from build123d import *

# Parameters (mm, degrees)
BOSS_EXTRUDE1_DEPTH     = 8.255
SKETCH2_R               = 9.525
BOSS_EXTRUDE2_DEPTH     = 0.635
CUT_EXTRUDE1_DEPTH      = 17.139496584
CUT_EXTRUDE1_DEPTH_BACK = 17.139496584
SKETCH3_R               = 2.159
FILLET1_R               = 2.54


with BuildPart() as part:
    # Sketch1 → Boss-Extrude1 (new body)
    with BuildSketch(Plane(origin=(0, 0, 0), x_dir=(1, 0, 0), z_dir=(0, 1, 0))):
        Polygon((7.18570145, 0), (3.592850725, 6.223), (-3.592850725, 6.223), (-7.18570145, 0), (-3.592850725, -6.223), (3.592850725, -6.223), align=None)
    extrude(amount=BOSS_EXTRUDE1_DEPTH)

    # Sketch2 → Boss-Extrude2 (add)
    with BuildSketch(Plane(origin=(0, 8.255, 0), x_dir=(1, 0, 0), z_dir=(0, 1, 0))):
        with Locations(Location((0, 0, 0), (0, 0, 270))):
            Circle(SKETCH2_R)
    extrude(amount=BOSS_EXTRUDE2_DEPTH)

    # Sketch3 → Cut-Extrude1 (cut, two sides: drawn at the far end of the back side and taken through both)
    with BuildSketch(Plane(origin=(0, 8.89, 0), x_dir=(1, 0, 0), z_dir=(0, 1, 0)).offset(-CUT_EXTRUDE1_DEPTH_BACK)):
        with Locations(Location((-4.064, 0, 0), (0, 0, 270))):
            Circle(SKETCH3_R)
        with Locations(Location((4.064, 0, 0), (0, 0, 270))):
            Circle(SKETCH3_R)
    extrude(amount=CUT_EXTRUDE1_DEPTH + CUT_EXTRUDE1_DEPTH_BACK, mode=Mode.SUBTRACT)

    # Fillet1
    fillet1_edges = [part.edges().sort_by_distance(p)[0] for p in [
        (3.592850725, 4.1275, 6.223),
        (-3.592850725, 4.1275, 6.223),
        (-7.18570145, 4.1275, 0),
        (-3.592850725, 4.1275, -6.223),
        (3.592850725, 4.1275, -6.223),
        (7.18570145, 4.1275, 0),
    ]]
    fillet(fillet1_edges, radius=FILLET1_R)


solid = part.part
The model under review builds one solid part; all positions refer to its coordinate system, in mm. A direction names the side the tool comes from. Coordinates: 2 decimals unless noted, no trailing zeros. Loops run counter-clockwise (first coordinate to the right, second up) from the corner with the lowest first, then second, coordinate; pieces in that order, holes last. Notation, with made-up numbers: M -14.5,40.5 L 39.5,40.5 A20 cw 39.5,62.5 Z; hole C 69,41 d6. An arc over 180 degrees is marked long. Put each result on its own line as item: value. Start each with the question number.
Q1. The part is to be moulded in two halves that separate along X. For faces 4 (the flat face through (-5.4, 4.07, 3.09)), 5 (the cylindrical face through (-2.244, 4.383, 1.161)), 6 (the flat face through (0, 0, 0)), 7 (the cylindrical face through (-5.796, 8.568, -7.559)), say which applies: +X half, -X half, draft (parallel to the pull), parting line (faces both ways), or undercut.
Q2. Wall thickness on line 1 (X direction, y = 6, z = 0) (3 decimals); line 2 (X direction, y = 1, z = 0.75); line 3 (Z direction, x = -4.25, y = 4.5): over which ranges is each line inside the solid? List them lowest first.
Q3. Add section D-D (y = 8). Write out the cut boundary in (x, z), and give its area (3 significant figures).
Q4. Add section C-C (z = -2.5). Write out the cut boundary in (x, y) (3 decimals).
Q5. Add section A-A (z = 0). Write out the cut boundary in (x, y) (3 decimals).
Q6. Add section B-B (x = 0). Write out the cut boundary in (y, z) (3 decimals).
Q7. For faces 1 (the cylindrical face through (3.38, 4.19, 5.89)), 2 (the cylindrical face through (-3.38, 4.19, -5.89)), 3 (the cylindrical face through (-6.793, 4.185, -0.019)), list the 3-axis set-ups (+Z, -Z, +X, -X, +Y, -Y) from which the entire face can be reached by the end or side of a thin tool; tool diameter is ignored.
Q8. Clearance check with flat-ended pins moving along their axes: pin 1 (3.5 mm diameter, centred on x = -4.064, z = 0, fed in from -Y); pin 2 (4 mm diameter, centred on x = 4.5, z = 4.5, fed in from -Y); pin 3 (5 mm diameter, centred on y = 5, z = 7, fed in from +X); pin 4 (4 mm diameter, centred on y = 7, z = -4.5, fed in from +X). State where each tip first meets the part, or that it passes through.
Answers:
1. face 4: -X half
1. face 5: undercut
1. face 6: draft
1. face 7: parting line
2. line 1: x = -6.793 to -6.223, -1.905 to 1.905, 6.223 to 6.793
2. line 2: x = -6.68 to -6.09, -2.04 to 2.04, 6.09 to 6.68
2. line 3: z = -5.08 to -2.15, 2.15 to 5.08
3. outline: M -6.45,-1.27 L -4.33,-4.95 A2.54 ccw -2.13,-6.22 L 2.13,-6.22 A2.54 ccw 4.33,-4.95 L 6.45,-1.27 A2.54 ccw 6.45,1.27 L 4.33,4.95 A2.54 ccw 2.13,6.22 L -2.13,6.22 A2.54 ccw -4.33,4.95 L -6.45,1.27 A2.54 ccw Z; hole C -4.06,0 d4.32; hole C 4.06,0 d4.32
3. area: 103 mm^2
4. outline: M -9.191,8.255 L -5.742,8.255 L -5.742,0 L 5.742,0 L 5.742,8.255 L 9.191,8.255 L 9.191,8.89 L -9.191,8.89 Z
5. outline: M -9.525,8.255 L -6.793,8.255 L -6.793,0 L -6.223,0 L -6.223,8.89 L -9.525,8.89 Z; M -1.905,0 L 1.905,0 L 1.905,8.89 L -1.905,8.89 Z; M 6.223,0 L 6.793,0 L 6.793,8.255 L 9.525,8.255 L 9.525,8.89 L 6.223,8.89 Z
6. outline: M 0,-6.223 L 8.255,-6.223 L 8.255,-9.525 L 8.89,-9.525 L 8.89,9.525 L 8.255,9.525 L 8.255,6.223 L 0,6.223 Z
7. face 1: +Z, +X, -Y
7. face 2: -Z, -X, -Y
7. face 3: -X, -Y
8. pin 1: passes through
8. pin 2: stops at y = 0
8. pin 3: stops at x = 4.59
8. pin 4: stops at x = 9.06
